Autodesk Inventor part; units mm, degrees
ref_plane "YZ Plane" through (0, 0, 0) normal (1, 0, 0) x (0, 1, 0)
ref_plane "XZ Plane" through (0, 0, 0) normal (0, 1, 0) x (-1, 0, 0)
ref_plane "XY Plane" through (0, 0, 0) normal (0, 0, 1) x (1, 0, 0)
sketch "Sketch1" plane through (0, 0, 0) normal (0, 0, 1) x (1, 0, 0)
  line L0 (-490, 40) -> (490, 40)
  line L1 (490, 40) -> (490, 0)
  line L2 (490, 0) -> (-490, 0)
  line L3 (-490, 0) -> (-490, 40)
  point P0 (0, 0)
  point P1 (0, 0)
  dimension "d0" = 980
  dimension "d1" = 40
extrude "Plate1" add sketch "Sketch1" along normal blind 2
sketch "Sketch2" plane through (490, 2, 0) normal (0, -1, 0) x (1, 0, 0)
  line L0 (-980, 0) -> (0, 0)
  line L1 (0, 0) -> (0, 20)
  line L2 (0, 20) -> (-980, 20)
  line L3 (-980, 20) -> (-980, 0)
edge flange "Flange1" height 20 angle 90 thickness 2 bend radius 2.75 thickness toward (0, -1, 0) relief round relief width 2 relief depth 1 edges at (0, 0, 2) wall of the first edge with corners at (-490, 2, 0) (490, 2, 0) (490, 2, 20) (-490, 2, 20)
bend "Bend1"
corner "Corner1"
sketch "Sketch9" plane through (0, 0, 2) normal (0, 0, 1) x (1, 0, 0)
  line L0 (-490, 4.75) -> (490, 4.75)
  line L1 (490, 40) -> (490, 4.75)
  line L2 (-490, 40) -> (490, 40)
  line L3 (-490, 4.75) -> (-490, 40)
  line L4 (0, 0) -> (0, 40) construction
  circle A0 centre (0, 40) radius 35
  circle A1 centre (490, 40) radius 35
  circle A2 centre (-490, 40) radius 35
  line L5 (246.05, 40) -> (243.95, 40)
  line L6 (243.95, 40) -> (243.95, 29)
  line L7 (243.95, 29) -> (246.05, 29)
  line L8 (246.05, 29) -> (246.05, 40)
  line L9 (-490, 40) -> (490, 40)
  line L10 (-246.05, 40) -> (-243.95, 40)
  line L11 (-243.95, 40) -> (-243.95, 29)
  line L12 (-243.95, 29) -> (-246.05, 29)
  line L13 (-246.05, 29) -> (-246.05, 40)
  line L14 (-490, 0) -> (490, 0)
  point P0 (-245, 29)
  point P1 (245, 29)
  point P2 (-243.95, 40)
  point P3 (-246.05, 40)
  point P4 (7.2068, 4.75)
  point P5 (35, 40)
  point P6 (-35, 40)
  point P7 (-7.2068, 4.75)
  point P8 (455, 40)
  point P9 (482.7932, 4.75)
  point P10 (-482.7932, 4.75)
  point P11 (-455, 40)
  point P12 (-490, 5)
  dimension "d41" = 70
  dimension "d42" = 490
  dimension "d43" = 2.1
  dimension "d44" = 29
  dimension "d45" = 11
extrude "Extrusion4" cut sketch "Sketch9" along normal through all both and the other way through all contours L3 A2 L2 L13 L12 L11 A0 L6 L7 L8 A1 L1 L0 | A2 L2 L3 | L3 L2 A2 | A1 L2 L1 | L2 L11 L12 L13 | L8 L7 L6 L2 | A0 L2 | L2 A0 picked at (473.6046, 23.6046)
sketch "Sketch10" plane through (0, 0, 2) normal (0, 0, 1) x (1, 0, 0)
  line L0 (483.1891, 23.5318) -> (483.1891, 11.5318) construction
  line L1 (483.1891, 11.5318) -> (283.1891, 11.5318) construction
  line L2 (283.1891, 11.5318) -> (283.1891, 23.5318) construction
  line L3 (283.1891, 23.5318) -> (483.1891, 23.5318) construction
  point P0 (0, 0)
  dimension "d48" = 200
  dimension "d49" = 12
feature "Mark2" [suppressed]
sketch "Sketch11" plane through (-490, 0, 20) normal (0, -1, 0) x (1, 0, 0)
  line L0 (0, -15.25) -> (0, -20)
  line L1 (0, 0) -> (980, 0)
  line L2 (0, -20) -> (778.54, -20)
  line L3 (778.54, -20) -> (778.54, 0)
  line L4 (778.54, 0) -> (0, 0)
  line L5 (0, 0) -> (0, -20)
  line L6 (778.54, 0) -> (754.7049, -20)
  line L7 (980, -20) -> (497.2068, -20)
  dimension "d50" = 778.54
  dimension "d51" = 50
extrude "Extrusion5" cut sketch "Sketch11" against normal through all contours L5 L1 L6 L2 L0
equation "\"d1\" = БОРТ_стрингер_4_высота"
equation "\"d2\" = Thickness"
equation "\"d3\" = BendReliefWidth"
equation "\"d4\" = BendReliefDepth"
equation "\"d5\" = MinimumRemnant"
equation "\"d6\" = TransitionRadius"
equation "\"d9\" = BendRadius"
equation "\"d10\" = CornerReliefSize"
equation "\"d11\" = GapSize"
equation "\"d12\" = JacobiRadiusSize"
equation "\"BendReliefWidth\" = Thickness"
equation "\"BendReliefDepth\" = 0.5 * Thickness"
equation "\"CornerReliefSize\" = 4 * Thickness"
equation "\"MinimumRemnant\" = 2 * Thickness"
equation "\"TransitionRadius\" = BendRadius"
equation "\"JacobiRadiusSize\" = BendRadius"
equation "\"GapSize\" = Thickness"
properties part number "MSC 328 STRINGER BOARD ##" material "Stainless Steel"
Can you work these out from the model? Positions are in its coordinate system, mm. A direction names the side the tool comes from. Coordinates: 2 decimals unless noted, no trailing zeros. Loops run counter-clockwise (first coordinate to the right, second up) from the corner with the lowest first, then second, coordinate; pieces in that order, holes last. Notation, with made-up numbers: M 26.25,28 L 36.25,28 A7 cw 36.25,37 Z; hole C -2.75,57.5 d8. An arc over 180 degrees is marked long. Return JSON: item names as keys, results as strings. Group by question number.
Item 1: Imagine slicing it at C-C (x = 279). Please give me the cut outline in (y, z) (3 decimals), and give its area (3 significant figures).
Item 2: Imagine slicing it at A-A (x = 348.5). Please give me the cut outline in (y, z), and give its area (3 significant figures).
Item 3: On a 3-axis mill with a long thin cutter (end or side, diameter ignored), from which of +Z, -Z, +X, -X, +Y, -Y can I reach the whole of each face in a straight line? I mean faces 1 (the flat face through (382, 0, 12)), 2 (the flat face through (382, 2, 12)). Say none if no direction works.
Item 4: If I drill on L1, parallel to Y at x = 347.5, z = 10.5; L2, parallel to Z at x = 398, y = 3.55; L3, parallel to Y at x = 374.5, z = 3.75, over which ranges is the centre line in solid material (lowest first)? Write a range as from..to.
Item 5: I'm going to push flat-ended pins straight in: pin 1 Ø1.5 at (x, y) = (429, 3.5) entering from +Z; pin 2 Ø2 at (y, z) = (1, 14.5) entering from -X; pin 3 Ø5 at (x, z) = (400, 7.5) entering from +Y. Where does each tip first touch, or does it pass through?
Item 6: Imagine slicing it at B-B (z = 16.5). Please give me the cut outline in (x, y).
Verdict:
{
 "1": {"outline": "M 0,4.75 A4.75 ccw 4.75,0 L 4.75,2 A2.75 cw 2,4.75 L 2,11.995 L 0,11.995 Z", "area": "26.3 mm^2"},
 "2": {"outline": "M 0,4.75 A4.75 ccw 4.75,0 L 4.75,2 A2.75 cw 2,4.75 L 2,20 L 0,20 Z", "area": "42.3 mm^2"},
 "3": {"face 1": "+Z, -Z, +X, -X, -Y", "face 2": "+Z, +X, -X, +Y"},
 "4": {"L1": "y = 0..2", "L2": "z = 0.15..2.28", "L3": "y = 0.11..2.19"},
 "5": {"pin 1": "stops at z = 2.86", "pin 2": "stops at x = 280.79", "pin 3": "stops at y = 2"},
 "6": {"outline": "M 284.37,0 L 490,0 L 490,2 L 284.37,2 Z"}
}
